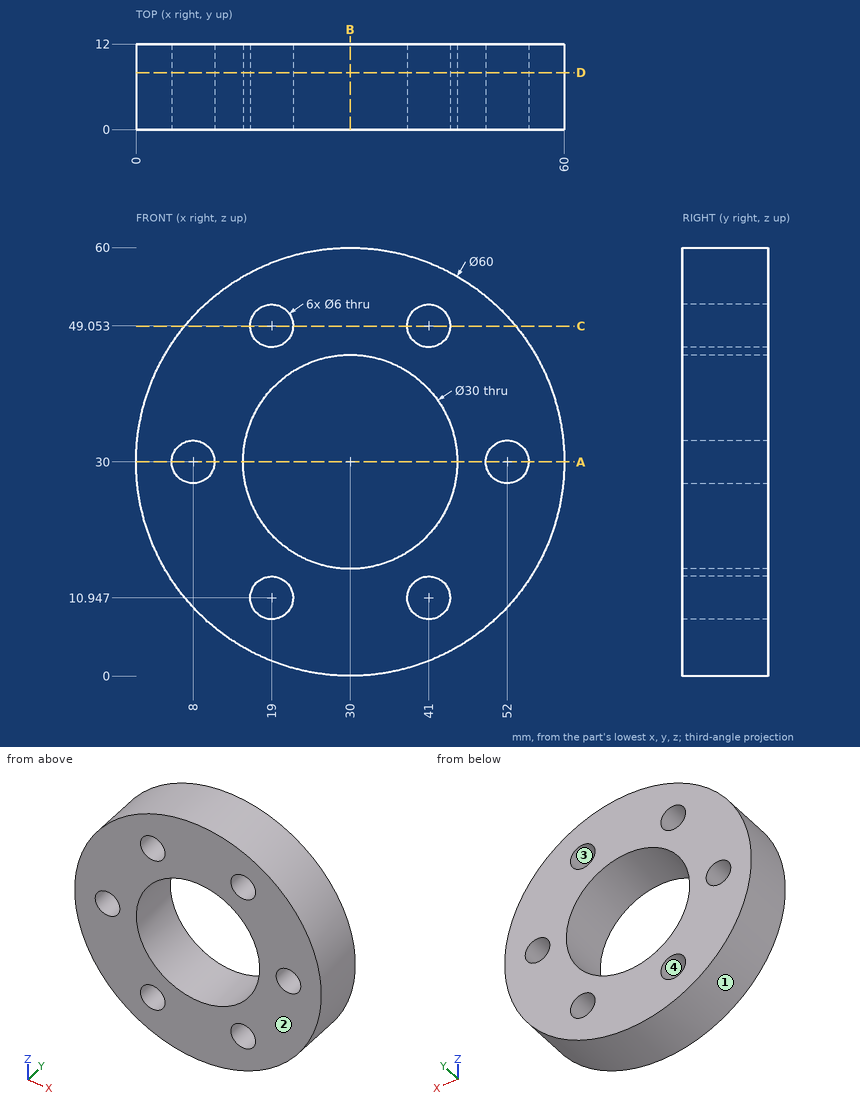
Geometry: see drawing. Coordinates: mm, zero at the bounding-box minimum. Round coordinates to 2 decimals unless told otherwise and drop trailing zeros. Loops run counter-clockwise (first coordinate to the right, second up) from the corner with the lowest first, then second, coordinate; pieces in that order, holes last. Notation, with made-up numbers: (12.5, 47.25) - (26.5, 47.25) arc R22 ccw to (26.5, 58.25) - close; hole circle Ø10 at (60.25, 41.5). An arc over 180 degrees is marked (long way). Use CSV: the item, a comma, the result in double quotes.
Q1. Section query C-C, the plane z = 49. Output: boundary loops of the cut face in (x, y).
Reported:
outline,"(6.78, 0) - (16, 0) - (16, 12) - (6.78, 12) - close; (22, 0) - (38, 0) - (38, 12) - (22, 12) - close; (44, 0) - (53.22, 0) - (53.22, 12) - (44, 12) - close"
Q2. Section query A-A, the plane z = 30. Output: boundary loops of the cut face in (x, y), then the cut area to 3 significant figures.
Reported:
outline,"(0, 0) - (5, 0) - (5, 12) - (0, 12) - close; (11, 0) - (15, 0) - (15, 12) - (11, 12) - close; (45, 0) - (49, 0) - (49, 12) - (45, 12) - close; (55, 0) - (60, 0) - (60, 12) - (55, 12) - close"
area,"216 mm^2"
Q3. Pin query (flat end, axial travel): pin 1 Ø2 at (y, z) = (8.5, 53.5) entering from -X (1 decimal); pin 2 Ø4 at (y, z) = (5.5, 27) entering from -X; pin 3 Ø6 at (y, z) = (9.5, 38.5) entering from +X. Return the tip coordinate at first contact, or that it passes through.
Reported:
pin 1,"x = 10.2"
pin 2,"x = 0.02"
pin 3,"x = 59.49"
Q4. Section query D-D, the plane y = 8. Output: boundary loops of the cut face in (x, z).
Reported:
outline,"circle Ø60 at (30, 30); hole circle Ø6 at (8, 30); hole circle Ø30 at (30, 30); hole circle Ø6 at (19, 10.95); hole circle Ø6 at (19, 49.05); hole circle Ø6 at (41, 10.95); hole circle Ø6 at (41, 49.05); hole circle Ø6 at (52, 30)"
Q5. Section query B-B, the plane x = 30. Output: boundary loops of the cut face in (y, z), then the cut area to 3 significant figures.
Reported:
outline,"(0, 0) - (12, 0) - (12, 15) - (0, 15) - close; (0, 45) - (12, 45) - (12, 60) - (0, 60) - close"
area,"360 mm^2"
Q6. Mould query, pull axis Z, two halves, no side actions, for the marked faces 1, 2, 3 and 4. Classes: pulls with the +Z half, pulls with the -Z half, needs draft (parallel to the pull), parting line crosses it, or undercut.
Reported:
face 1,"parting line crosses it"
face 2,"needs draft"
face 3,"undercut"
face 4,"undercut"
Q7. Ray query, line 1 along X through (y, z) = (4.25, 30); line 2 along X through (y, z) = (3.5, 10) (1 decimal); line 3 along Z through (x, y) = (16.5, 9.5) (1 decimal). Return the intervals inside material, ascending.
Reported:
line 1,"0 to 5, 11 to 15, 45 to 49, 55 to 60"
line 2,"7.6 to 16.2, 21.8 to 38.2, 43.8 to 52.4"
line 3,"3.2 to 9.3, 12.6 to 23.5, 36.5 to 47.4, 50.7 to 56.8"
